```python
from build123d import *

# Parameters (mm, degrees)
SKETCH_1_R          = 9.5
EXTRUDE_2_DEPTH     = 73
EXTRUDE_START       = -3
EXTRUDE_3_DEPTH     = 3
EXTRUDE_4_DEPTH     = 3
EXTRUDE_5_DEPTH     = 3
EXTRUDE_6_DEPTH     = 3
SKETCH_8_W          = 3
SKETCH_8_H          = 6.1
EXTRUDE_7_DEPTH     = 12.1
SKETCH_9_W          = 3
SKETCH_9_H          = 6.1
EXTRUDE_8_DEPTH     = 12.1
SKETCH_10_W         = 3
SKETCH_10_H         = 5
EXTRUDE_9_DEPTH     = 12.1
SKETCH_11_W         = 3
SKETCH_11_H         = 5
EXTRUDE_10_DEPTH    = 12.1
EXTRUDE_11_DEPTH    = 3
EXTRUDE_12_DEPTH    = 3
EXTRUDE_13_DEPTH    = 3
EXTRUDE_14_DEPTH    = 3
EXTRUDE_15_DEPTH    = 6.1
SKETCH_18_W         = 13.5
SKETCH_18_H         = 6
EXTRUDE_16_DEPTH    = 2
EXTRUDE_START_2     = -2
SKETCH_19_W         = 13.5
SKETCH_19_H         = 6
EXTRUDE_17_DEPTH    = 2
SKETCH_20_W         = 13.5
SKETCH_20_H         = 2
EXTRUDE_18_DEPTH    = 12.5
EXTRUDE_START_3     = -10
EXTRUDE_19_DEPTH    = 10
EXTRUDE_20_DEPTH    = 10
EXTRUDE_START_4     = 36.5
EXTRUDE_21_DEPTH    = 5
CUT_EXTRUDE_1_DEPTH = 5


with BuildPart() as part:
    # Sketch 1 → Extrude 2 (new body)
    with BuildSketch(Plane.XY):
        with BuildLine():
            Line((-28.056349186, -15.556349186), (-28.056349186, -28.056349186))
            Line((-28.056349186, -28.056349186), (-15.556349186, -28.056349186))
            ThreePointArc((-15.556349186, -28.056349186), (-6.717514421, -24.395183951), (-3.056349186, -15.556349186))
            Line((-3.056349186, -15.556349186), (3.056349186, -15.556349186))
            ThreePointArc((3.056349186, -15.556349186), (17.365374305, -27.924753615), (27.532737685, -11.976388499))
            ThreePointArc((27.532737685, -11.976388499), (41.137654945, 7.466608715), (18.612698372, 0))
            Line((18.612698372, 0), (12.5, 0))
            ThreePointArc((12.5, 0), (-1.809025119, 12.368404429), (-11.976388499, -3.579960687))
            ThreePointArc((-11.976388499, -3.579960687), (-23.022957901, -5.531392613), (-28.056349186, -15.556349186))
        make_face()
        with Locations((-15.556349186, -15.556349186)):
            Circle(SKETCH_1_R, mode=Mode.SUBTRACT)
        with Locations((15.556349186, -15.556349186)):
            Circle(SKETCH_1_R, mode=Mode.SUBTRACT)
        Circle(SKETCH_1_R, mode=Mode.SUBTRACT)
        with Locations((31.112698372, 0)):
            Circle(SKETCH_1_R, mode=Mode.SUBTRACT)
    extrude(amount=EXTRUDE_2_DEPTH)

    # Sketch 4 → Extrude 3 (add)
    with BuildSketch(Plane.XY.offset(61.05).offset(EXTRUDE_START)):
        with BuildLine():
            ThreePointArc((-12.229391425, 2.586887198), (-10.355088747, 7.001581039), (-6.956349186, 10.385528682))
            Line((-6.956349186, 10.385528682), (-6.956349186, 22.043650814))
            Line((-6.956349186, 22.043650814), (-23.056349186, 22.043650814))
            Line((-23.056349186, 22.043650814), (-23.056349186, 15.943650814))
            ThreePointArc((-23.056349186, 15.943650814), (-15.231128181, 12.702338145), (-11.989815512, 4.87711714))
            ThreePointArc((-11.989815512, 4.87711714), (-12.049872452, 3.725753839), (-12.229391425, 2.586887198))
        make_face()
    extrude(amount=EXTRUDE_3_DEPTH)

    # Sketch 5 → Extrude 4 (add)
    with BuildSketch(Plane.XY.offset(11.95)):
        with BuildLine():
            ThreePointArc((-12.229391425, 2.586887198), (-10.355088747, 7.001581039), (-6.956349186, 10.385528682))
            Line((-6.956349186, 10.385528682), (-6.956349186, 22.043650814))
            Line((-6.956349186, 22.043650814), (-23.056349186, 22.043650814))
            Line((-23.056349186, 22.043650814), (-23.056349186, 15.943650814))
            ThreePointArc((-23.056349186, 15.943650814), (-15.231128181, 12.702338145), (-11.989815512, 4.87711714))
            ThreePointArc((-11.989815512, 4.87711714), (-12.049872452, 3.725753839), (-12.229391425, 2.586887198))
        make_face()
    extrude(amount=EXTRUDE_4_DEPTH)

    # Sketch 7 → Extrude 6 (add)
    with BuildSketch(Plane.XY.offset(30.05).offset(EXTRUDE_START)):
        with BuildLine():
            ThreePointArc((-12.229391425, 2.586887198), (-10.355088747, 7.001581039), (-6.956349186, 10.385528682))
            Line((-6.956349186, 10.385528682), (-6.956349186, 22.043650814))
            Line((-6.956349186, 22.043650814), (-23.056349186, 22.043650814))
            Line((-23.056349186, 22.043650814), (-23.056349186, 15.943650814))
            ThreePointArc((-23.056349186, 15.943650814), (-15.231128181, 12.702338145), (-11.989815512, 4.87711714))
            ThreePointArc((-11.989815512, 4.87711714), (-12.049872452, 3.725753839), (-12.229391425, 2.586887198))
        make_face()
    extrude(amount=EXTRUDE_6_DEPTH)

    # Sketch 8 → Extrude 7 (add)
    with BuildSketch(Plane.XY.offset(14.95)):
        with Locations((-21.556349186, 18.993650814)):
            Rectangle(SKETCH_8_W, SKETCH_8_H)
    extrude(amount=EXTRUDE_7_DEPTH)



with BuildPart() as body_2:
    # Sketch 6 → Extrude 5 (new body)
    with BuildSketch(Plane.XY.offset(42.95)):
        with BuildLine():
            ThreePointArc((-12.229391425, 2.586887198), (-10.355088747, 7.001581039), (-6.956349186, 10.385528682))
            Line((-6.956349186, 10.385528682), (-6.956349186, 22.043650814))
            Line((-6.956349186, 22.043650814), (-23.056349186, 22.043650814))
            Line((-23.056349186, 22.043650814), (-23.056349186, 15.943650814))
            ThreePointArc((-23.056349186, 15.943650814), (-15.231128181, 12.702338145), (-11.989815512, 4.87711714))
            ThreePointArc((-11.989815512, 4.87711714), (-12.049872452, 3.725753839), (-12.229391425, 2.586887198))
        make_face()
    extrude(amount=EXTRUDE_5_DEPTH)


with BuildPart() as part_1:
    add(part.part)

    add(body_2.part)  # Extrude 8 merges body 2
    # Sketch 9 → Extrude 8 (add)
    with BuildSketch(Plane.XY.offset(45.95)):
        with Locations((-21.556349186, 18.993650814)):
            Rectangle(SKETCH_9_W, SKETCH_9_H)
    extrude(amount=EXTRUDE_8_DEPTH)

    # Sketch 10 → Extrude 9 (add)
    with BuildSketch(Plane.XY.offset(45.95)):
        with Locations((-8.456349186, 19.543650814)):
            Rectangle(SKETCH_10_W, SKETCH_10_H)
    extrude(amount=EXTRUDE_9_DEPTH)

    # Sketch 11 → Extrude 10 (add)
    with BuildSketch(Plane(origin=(0, 0, 27.05), x_dir=(-1, 0, 0), z_dir=(0, 0, -1))):
        with Locations((8.456349186, 19.543650814)):
            Rectangle(SKETCH_11_W, SKETCH_11_H)
    extrude(amount=EXTRUDE_10_DEPTH)

    # Sketch 12 → Extrude 11 (add)
    with BuildSketch(Plane(origin=(0, 0, 11.95), x_dir=(-1, 0, 0), z_dir=(0, 0, -1))):
        with BuildLine():
            Line((6.956349186, 10.385528682), (6.956349186, 12.89295364))
            ThreePointArc((6.956349186, 12.89295364), (6.284928313, 11.642571046), (4.871740345, 11.51156575))
            ThreePointArc((4.871740345, 11.51156575), (5.940784069, 10.998049129), (6.956349186, 10.385528682))
        make_face()
    extrude(amount=-EXTRUDE_11_DEPTH)

    # Sketch 13 → Extrude 12 (add)
    with BuildSketch(Plane(origin=(0, 0, 27.05), x_dir=(-1, 0, 0), z_dir=(0, 0, -1))):
        with BuildLine():
            Line((6.956349186, 10.385528682), (6.956349186, 12.89295364))
            ThreePointArc((6.956349186, 12.89295364), (6.284928313, 11.642571046), (4.871740345, 11.51156575))
            ThreePointArc((4.871740345, 11.51156575), (5.940784069, 10.998049129), (6.956349186, 10.385528682))
        make_face()
    extrude(amount=-EXTRUDE_12_DEPTH)

    # Sketch 14 → Extrude 13 (add)
    with BuildSketch(Plane(origin=(0, 0, 42.95), x_dir=(-1, 0, 0), z_dir=(0, 0, -1))):
        with BuildLine():
            Line((6.956349186, 10.385528682), (6.956349186, 12.89295364))
            ThreePointArc((6.956349186, 12.89295364), (6.284928313, 11.642571046), (4.871740345, 11.51156575))
            ThreePointArc((4.871740345, 11.51156575), (5.940784069, 10.998049129), (6.956349186, 10.385528682))
        make_face()
    extrude(amount=-EXTRUDE_13_DEPTH)

    # Sketch 15 → Extrude 14 (add)
    with BuildSketch(Plane(origin=(0, 0, 58.05), x_dir=(-1, 0, 0), z_dir=(0, 0, -1))):
        with BuildLine():
            Line((6.956349186, 10.385528682), (6.956349186, 12.89295364))
            ThreePointArc((6.956349186, 12.89295364), (6.284928313, 11.642571046), (4.871740345, 11.51156575))
            ThreePointArc((4.871740345, 11.51156575), (5.940784069, 10.998049129), (6.956349186, 10.385528682))
        make_face()
    extrude(amount=-EXTRUDE_14_DEPTH)

    # Sketch 16 → Extrude 15 (add)
    with BuildSketch(Plane.XZ.offset(-22.043650814)):
        Polygon((-23.056349186, 18.75), (-23.056349186, 23.25), (-26.056349186, 25), (-26.056349186, 17), align=None)
        Polygon((-23.056349186, 49.75), (-23.056349186, 54.25), (-26.056349186, 56), (-26.056349186, 48), align=None)
    extrude(amount=EXTRUDE_15_DEPTH)

    # Sketch 18 → Extrude 16 (add)
    with BuildSketch(Plane.XY.offset(42.75)):
        with BuildLine():
            Line((13.237836074, 16.043650814), (-0.262163926, 16.043650814))
            Line((-0.262163926, 16.043650814), (-0.262163926, 12.497250501))
            ThreePointArc((-0.262163926, 12.497250501), (8.745654662, 8.931042746), (12.5, 0))
            Line((12.5, 0), (18.612698372, 0))
            ThreePointArc((18.612698372, 0), (20.996031333, 7.341869518), (27.237186055, 11.884039897))
            ThreePointArc((27.237186055, 11.884039897), (17.647498042, 13.394958805), (13.237836074, 22.043650814))
            Line((13.237836074, 22.043650814), (13.237836074, 16.043650814))
        make_face()
        with Locations((6.487836074, 19.043650814)):
            Rectangle(SKETCH_18_W, SKETCH_18_H)
    extrude(amount=EXTRUDE_16_DEPTH)

    # Sketch 19 → Extrude 17 (add)
    with BuildSketch(Plane.XY.offset(30.25).offset(EXTRUDE_START_2)):
        with BuildLine():
            Line((13.237836074, 16.043650814), (-0.262163926, 16.043650814))
            Line((-0.262163926, 16.043650814), (-0.262163926, 12.497250501))
            ThreePointArc((-0.262163926, 12.497250501), (8.745654662, 8.931042746), (12.5, 0))
            Line((12.5, 0), (18.612698372, 0))
            ThreePointArc((18.612698372, 0), (20.996031333, 7.341869518), (27.237186055, 11.884039897))
            ThreePointArc((27.237186055, 11.884039897), (17.647498042, 13.394958805), (13.237836074, 22.043650814))
            Line((13.237836074, 22.043650814), (13.237836074, 16.043650814))
        make_face()
        with Locations((6.487836074, 19.043650814)):
            Rectangle(SKETCH_19_W, SKETCH_19_H)
    extrude(amount=EXTRUDE_17_DEPTH)

    # Sketch 20 → Extrude 18 (add)
    with BuildSketch(Plane(origin=(0, 0, 42.75), x_dir=(-1, 0, 0), z_dir=(0, 0, -1))):
        with Locations((-6.487836074, 15.043650814)):
            Rectangle(SKETCH_20_W, SKETCH_20_H)
    extrude(amount=EXTRUDE_18_DEPTH)

    # Sketch 22 → Extrude 19 (add)
    with BuildSketch(Plane.XY.offset(73).offset(EXTRUDE_START_3)):
        with BuildLine():
            Line((31.112698372, 12.5), (43.612698372, 12.5))
            Line((43.612698372, 12.5), (43.612698372, 0))
            ThreePointArc((43.612698372, 0), (39.951533137, 8.838834765), (31.112698372, 12.5))
        make_face()
    extrude(amount=EXTRUDE_19_DEPTH)

    # Sketch 23 → Extrude 20 (add)
    with BuildSketch(Plane.XY):
        with BuildLine():
            Line((43.612698372, 12.5), (31.112698372, 12.5))
            ThreePointArc((31.112698372, 12.5), (39.951533137, 8.838834765), (43.612698372, 0))
            Line((43.612698372, 0), (43.612698372, 12.5))
        make_face()
    extrude(amount=EXTRUDE_20_DEPTH)

    # Sketch 24 → Extrude 21 (add, symmetric)
    with BuildSketch(Plane.XY.offset(EXTRUDE_START_4)):
        with BuildLine():
            Line((43.612698372, 12.5), (31.112698372, 12.5))
            ThreePointArc((31.112698372, 12.5), (39.951533137, 8.838834765), (43.612698372, 0))
            Line((43.612698372, 0), (43.612698372, 12.5))
        make_face()
    extrude(amount=EXTRUDE_21_DEPTH, both=True)

    # Sketch 25 → Cut-Extrude 1 (cut)
    with BuildSketch(Plane(origin=(0, 12.5, 0), x_dir=(1, 0, 0), z_dir=(0, 1, 0))):
        Polygon((43.612698372, -65.75), (40.612698372, -64), (40.612698372, -72), (43.612698372, -70.25), align=None)
        Polygon((40.612698372, -32.5), (43.612698372, -34.25), (43.612698372, -38.75), (40.612698372, -40.5), align=None)
        Polygon((43.612698372, -2.75), (43.612698372, -7.25), (40.612698372, -9), (40.612698372, -1), align=None)
    extrude(amount=-CUT_EXTRUDE_1_DEPTH, mode=Mode.SUBTRACT)


solid = part_1.part
```
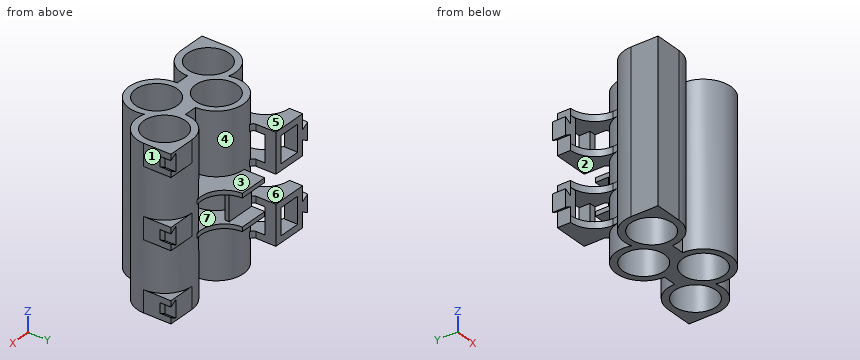
Design review of the part built by this model. Coordinates are the model's own, in mm. Face numbers are marked on the shaded views. A direction names the side the tool comes from. Give positions to 0.01 mm unless a question says otherwise; leave off trailing zeros. Write each loop counter-clockwise with the first axis right and the second up, starting at its lowest first coordinate (ties: lowest second). Pieces come first, ordered by that corner, then holes.
(1) Clearance check with flat-ended pins moving along their axes: pin 1 Ø12 at (x, z) = (8, 58.5) entering from -Y; pin 2 Ø20 at (x, y) = (-16.5, 9.5) entering from -Z; pin 3 Ø6 at (x, z) = (8.5, 33.5) entering from -Y; pin 4 Ø1.5 at (y, z) = (9, 5) entering from +X. State where each tip first meets the part, or that it passes through.
Checked values:
pin 1: stops at y = -27.96
pin 2: stops at z = 0
pin 3: stops at y = -27.38
pin 4: stops at x = 40.61
(2) Tool access review of the marked faces 5, 6 and 7: name each direction out of +Z, -Z, +X, -X, +Y, -Y from which nothing blocks a thin tool from reaching the whole face with its end or side.
Checked values:
face 5: +Z, -X, +Y
face 6: -X, +Y
face 7: none
(3) Mouldability with a two-part tool opening along Z and no side actions: class the marked faces 1, 2, 3 and 4 as +Z half, -Z half, draft (parallel to the pull), parting line (faces both ways), or undercut.
Checked values:
face 1: draft
face 2: undercut
face 3: +Z half
face 4: undercut
(4) Add section B-B (y = 15). Give the boundary of the cut face in (x, z), and give its area (3 significant figures).
Checked values:
outline: (-18.58, 11.95) - (-6.96, 11.95) - (-6.96, 14.95) - (-18.58, 14.95) - close; (-18.58, 27.05) - (-6.96, 27.05) - (-6.96, 30.05) - (-18.58, 30.05) - close; (-18.58, 42.95) - (-6.96, 42.95) - (-6.96, 45.95) - (-18.58, 45.95) - close; (-18.58, 58.05) - (-6.96, 58.05) - (-6.96, 61.05) - (-18.58, 61.05) - close; (-0.26, 28.25) - (15.89, 28.25) - (15.89, 30.25) - (13.24, 30.25) - (13.24, 42.75) - (15.89, 42.75) - (15.89, 44.75) - (-0.26, 44.75) - close
area: 373 mm2
(5) Wall thickness on line 1 along Y through (x, z) = (31.5, 25.5); line 2 along X through (y, z) = (-15.5, 46); line 3 along X through (y, z) = (-20.5, 61): over which ranges is each line inside the solid? List them lowest first.
Checked values:
line 1: y = -12.49 to -9.49, 9.49 to 12.49
line 2: x = -28.06 to -25.06, -6.06 to 6.06, 25.06 to 28.06
line 3: x = -28.06 to -23.67, -7.44 to -4.08, 4.08 to 7.44, 23.67 to 27.04
(6) Add section C-C (z = 5). Give the boundary of the cut face in (x, y).
Checked values:
outline: (-28.06, -28.06) - (-15.56, -28.06) arc R12.5 ccw to (-3.06, -15.56) - (3.06, -15.56) arc R12.5 ccw (long way) to (27.53, -11.98) arc R12.5 ccw to (43.61, 0) - (43.61, 7.5) - (40.61, 7.5) - (40.61, 12.5) - (31.11, 12.5) arc R12.5 ccw to (18.61, 0) - (12.5, 0) arc R12.5 ccw (long way) to (-11.98, -3.58) arc R12.5 ccw to (-28.06, -15.56) - close; hole circle Ø19 at (-15.56, -15.56); hole circle Ø19 at (0, 0); hole circle Ø19 at (15.56, -15.56); hole circle Ø19 at (31.11, 0)
(7) Add section A-A (x = 29). Give the boundary of the cut face in (y, z).
Checked values:
outline: (-12.32, 0) - (-9.26, 0) - (-9.26, 73) - (-12.32, 73) - close; (9.26, 0) - (12.32, 0) - (12.32, 73) - (9.26, 73) - close
